Model file for the job. Use its own axes, mm. Face numbers are marked on the shaded views. A direction names the side the tool comes from. Coordinates: 2 decimals unless noted, no trailing zeros. Write each loop counter-clockwise with the first axis right and the second up, starting at its lowest first coordinate (ties: lowest second). Pieces come first, ordered by that corner, then holes. Notation, with made-up numbers: M -18.5,42.25 L -0.5,42.25 A37 cw -0.5,78.25 Z; hole C -32,-37 d3. An arc over 180 degrees is marked long. Put each result on its own line as item: value. Start each with the question number.
Q1. Cut at D-D (y = 0.35). Write the cut outline in (x, z).
Q2. Cut at A-A (z = 0). Write the cut outline in (x, y), then the cut area to 3 significant figures.
Q3. Cut at B-B (x = 20). Write the cut outline in (y, z).
Q4. Drill centre lines: line 1 along Z through (x, y) = (18, 1.5); line 2 along X through (y, z) = (0.85, 0.5); line 3 along X through (y, z) = (0.35, -13.25). Where is each one in solid material? Low to high.
Q5. Drop flat-ended pins along their axis: pin 1 (8 mm diameter, centred on x = 10.5, z = -6.5, fed in from -Y); pin 2 (0.6 mm diameter, centred on x = 22, y = 0.5, fed in from +Z); pin 3 (1 mm diameter, centred on x = 18, y = 1, fed in from -Z); pin 4 (1 mm diameter, centred on y = 1.5, z = -11.5, fed in from +X). Give the stop position or say it passes through.
Q6. Which spindle directions (+Z, -Z, +X, -X, +Y, -Y) get a long thin tool onto all of the face, cutting with end or side? Do the marked faces 1, 2 and 3. Say none if no direction does.
Q7. Pull direction Z, two halves, no side cores. Call the marked faces 4, 5, 6 and 7: pulls with the +Z half, pulls with the -Z half, needs draft (parallel to the pull), parting line crosses it, or undercut.
Q8. Cut at C-C (x = 13). Write the cut outline in (y, z).
```python
from build123d import *

# Parameters (mm, degrees)
SKETCH_1_R      = 1.15
EXTRUDE_1_DEPTH = 2
FILLET_1_R      = 6
FILLET_2_R      = 1.5


with BuildPart() as part:
    # Эскиз1 → Бобышка-Вытянуть1 (new body)
    with BuildSketch(Plane(origin=(0, 0, 0), x_dir=(1, 0, 0), z_dir=(0, 1, 0))):
        with BuildLine():
            Line((9.428338388, 13.219880501), (0.039848451, 2.999735338))
            ThreePointArc((0.039848451, 2.999735338), (-2.746686597, -1.206529212), (2.236067977, -2))
            Line((2.236067977, -2), (30.613932023, -2))
            ThreePointArc((30.613932023, -2), (35.722901746, -0.863965023), (32.087988444, 2.90160962))
            Line((32.087988444, 2.90160962), (15.382237716, 13.948474823))
            ThreePointArc((15.382237716, 13.948474823), (12.049527364, 16.491369305), (9.428338388, 13.219880501))
        make_face()
        with Locations(Location((0, 0, 0), (0, 0, 270))):
            Circle(SKETCH_1_R, mode=Mode.SUBTRACT)
        with Locations(Location((12.413926941, 13.513582719, 0), (0, 0, 270))):
            Circle(SKETCH_1_R, mode=Mode.SUBTRACT)
        Polygon((4.55303787, 2), (12.733176086, 10.904754713), (26.199495246, 2), align=None, mode=Mode.SUBTRACT)
    extrude(amount=EXTRUDE_1_DEPTH)

    # Скругление1
    fillet_1_edges = [part.edges().sort_by_distance(p)[0] for p in [
        (2.236067977, 1, 2),
        (0.039848451, 1, -2.999735338),
        (9.428338388, 1, -13.219880501),
        (15.382237716, 1, -13.948474823),
        (32.087988444, 1, -2.90160962),
        (30.613932023, 1, 2),
    ]]
    fillet(fillet_1_edges, radius=FILLET_1_R)

    # Скругление2
    fillet_2_edges = [part.edges().sort_by_distance(p)[0] for p in [
        (26.199495246, 1, -2),
        (12.733176086, 1, -10.904754713),
        (4.55303787, 1, -2),
    ]]
    fillet(fillet_2_edges, radius=FILLET_2_R)


solid = part.part
```
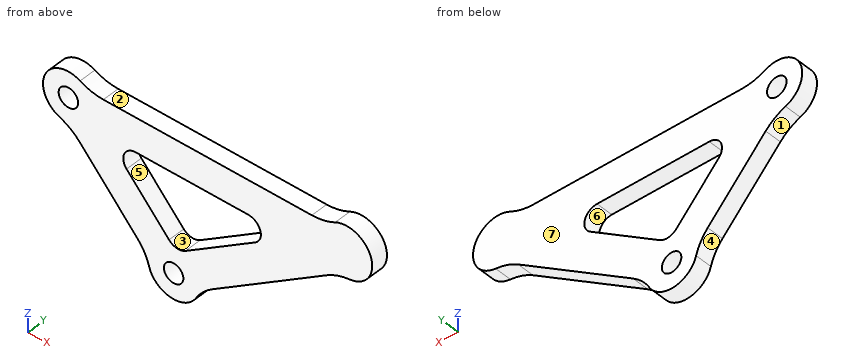
Computed values:
1. outline: M -1.03,-2.82 A6 cw 1.32,-4.39 L 8.15,-11.83 A6 cw 9.52,-14.31 A3 ccw 15.03,-14.98 A6 cw 16.96,-12.91 L 30.51,-3.94 A6 cw 33.17,-2.98 A3 ccw long 31.48,2.67 A6 cw 28.73,2 L 4.12,2 A6 cw 1.37,2.67 A3 ccw long Z; hole C 0,0 d2.3; hole M 6.86,-4.51 L 11.87,-9.96 A1.5 ccw 13.8,-10.2 L 22.04,-4.75 A1.5 ccw 21.21,-2 L 7.97,-2 A1.5 ccw Z; hole C 12.41,-13.51 d2.3
2. outline: M -3,0 L -1.15,0 L -1.15,2 L -3,2 Z; M 1.15,0 L 35.85,0 L 35.85,2 L 1.15,2 Z
2. area: 73.1 mm2
3. outline: M 0,-10.89 L 2,-10.89 L 2,-6.1 L 0,-6.1 Z; M 0,-2 L 2,-2 L 2,2 L 0,2 Z
4. line 1: -12.22 to -7.42, -2 to 2
4. line 2: -2.96 to -1.04, 1.04 to 35.81
4. line 3: 9.12 to 11.29, 13.53 to 16.49
5. pin 1: y = 0
5. pin 2: z = 2
5. pin 3: z = -12.55
5. pin 4: x = 19.84
6. face 1: -Z, -X, +Y, -Y
6. face 2: +Z, +Y, -Y
6. face 3: +Y, -Y
7. face 4: pulls with the -Z half
7. face 5: undercut
7. face 6: undercut
7. face 7: needs draft
8. outline: M 0,-16.46 L 2,-16.46 L 2,-14.5 L 0,-14.5 Z; M 0,-12.52 L 2,-12.52 L 2,-10.45 L 0,-10.45 Z; M 0,-2 L 2,-2 L 2,2 L 0,2 Z
